Autodesk Inventor part; units mm, degrees
ref_plane "YZ Plane" through (0, 0, 0) normal (1, 0, 0) x (0, 1, 0)
ref_plane "XZ Plane" through (0, 0, 0) normal (0, 1, 0) x (-1, 0, 0)
ref_plane "XY Plane" through (0, 0, 0) normal (0, 0, 1) x (1, 0, 0)
sketch "Sketch1" plane through (0, 0, 0) normal (0, 0, 1) x (1, 0, 0)
  circle A0 centre (3.9687, -260.35) radius 2.1844
  circle A1 centre (16.6687, -260.35) radius 2.1844
  circle A2 centre (3.9687, -6.35) radius 2.1844
  circle A3 centre (16.6687, -6.35) radius 2.1844
  line L0 (3.175, -266.7) -> (8.0073, -266.7)
  line L1 (12.6301, -266.7) -> (16.4968, -266.7)
  line L2 (41.8702, 0) -> (3.175, 0)
  line L3 (3.175, -266.7) -> (16.4968, -266.7)
  line L4 (45.0452, -238.4496) -> (45.0452, -3.175)
  line L5 (41.8702, 0) -> (3.175, 0)
  line L6 (0, -3.175) -> (0, -263.525)
  circle A4 centre (3.9687, -260.35) radius 2.1844
  circle A5 centre (16.6687, -260.35) radius 2.1844
  circle A6 centre (3.9687, -6.35) radius 2.1844
  circle A7 centre (16.6687, -6.35) radius 2.1844
  arc A8 (0, -263.525) -> (3.175, -266.7) centre (3.175, -263.525) ccw
  arc A9 (3.175, 0) -> (0, -3.175) centre (3.175, -3.175) ccw
  arc A10 (45.0452, -3.175) -> (41.8702, 0) centre (41.8702, -3.175) ccw
  line L7 (18.7286, -265.7833) -> (44.1019, -240.7079)
  arc A11 (16.4968, -266.7) -> (18.7286, -265.7833) centre (16.4968, -263.525) ccw
  arc A12 (44.1019, -240.7079) -> (45.0452, -238.4496) centre (41.8702, -238.4496) ccw
  point P0 (0, 0)
  point P1 (18.3752, -266.7)
  point P2 (19.0379, -265.4777)
  point P3 (21.2768, -266.7)
  point P4 (45.0452, -243.1716)
  point P5 (43.8497, -240.9572)
  dimension "d5" = 3.175
extrude "Extrusion1" add sketch "Sketch1" along normal blind 1.5875
properties part number "wingplexi"
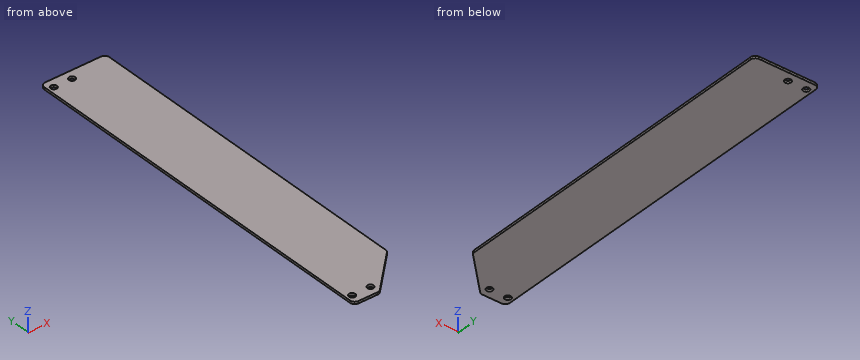
The model under review builds one solid part; all positions refer to its coordinate system, in mm. Round coordinates to 2 decimals unless told otherwise and drop trailing zeros. Write each loop counter-clockwise with the first axis right and the second up, starting at its lowest first coordinate (ties: lowest second). Pieces come first, ordered by that corner, then holes. Notation, with made-up numbers: (17.25, 19.5) - (74.25, 19.5) arc R32 cw to (74.25, 53.5) - close; hole circle Ø10 at (87.5, 48.5). An arc over 180 degrees is marked (long way). One line per question, with ' | ' between items.
Item 1: Add section B-B, the plane z = 0.55. Give the boundary of the cut face in (x, y) (3 decimals), then the cut area to 3 significant figures.
Resolved:
outline: (0, -263.525) arc R3.175 ccw to (3.175, -266.7) - (16.497, -266.7) arc R3.175 ccw to (18.729, -265.783) - (44.102, -240.708) arc R3.175 ccw to (45.045, -238.45) - (45.045, -3.175) arc R3.175 ccw to (41.87, 0) - (3.175, 0) arc R3.175 ccw to (0, -3.175) - close; hole circle Ø4.369 at (3.969, -260.35); hole circle Ø4.369 at (3.969, -6.35); hole circle Ø4.369 at (16.669, -260.35); hole circle Ø4.369 at (16.669, -6.35) | area: 11,600 mm2
Item 2: For P1, Ø3.5, axis at x = 16.67, y = -260.35, coming from the +Z side, flat-tipped, find the tip position at first contact; note if it passes through.
Resolved:
P1: passes through
Item 3: Add section C-C, the plane y = -260.35. Give the boundary of the cut face in (x, z), then the cut area to 3 significant figures.
Resolved:
outline: (0, 0) - (1.78, 0) - (1.78, 1.59) - (0, 1.59) - close; (6.15, 0) - (14.48, 0) - (14.48, 1.59) - (6.15, 1.59) - close; (18.85, 0) - (24.23, 0) - (24.23, 1.59) - (18.85, 1.59) - close | area: 24.6 mm2
Item 4: To check wall thickness, follow probe 1 along X at (y, z) = (-260.35, 0.95); probe 2 along Y at (x, z) = (28, 1); probe 3 along Y at (x, z) = (23.5, 0.4). State the ranges of each line that lie inside material, in increasing order.
Resolved:
probe 1: x = 0 to 1.78, 6.15 to 14.48, 18.85 to 24.23 | probe 2: y = -256.62 to 0 | probe 3: y = -261.07 to 0
Item 5: Add section D-D, the plane x = 34. Give the boundary of the cut face in (y, z).
Resolved:
outline: (-250.69, 0) - (0, 0) - (0, 1.59) - (-250.69, 1.59) - close
Item 6: Add section A-A, the plane y = -6.35. Give the boundary of the cut face in (x, z).
Resolved:
outline: (0, 0) - (1.78, 0) - (1.78, 1.59) - (0, 1.59) - close; (6.15, 0) - (14.48, 0) - (14.48, 1.59) - (6.15, 1.59) - close; (18.85, 0) - (45.05, 0) - (45.05, 1.59) - (18.85, 1.59) - close
